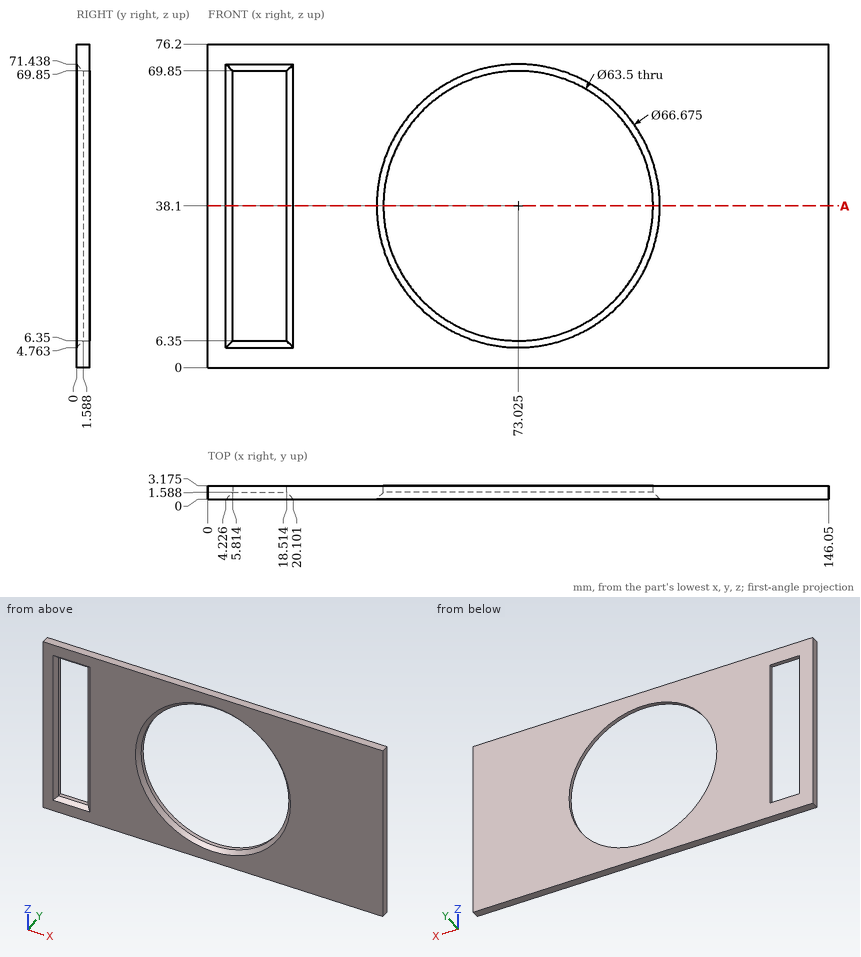
Answer from the drawing. Dimensions are ordinates in mm from the lowest x, y and z of the part. Coordinates: 2 decimals unless noted, no trailing zeros.
1) Section A-A (z = 38.1) is taken. Give the number of separate pieces and of enclosed holes in the cut face, plus the area to 3 significant figures.
Results:
separate pieces: 3
enclosed holes: 0
area: 217 mm2
2) Consider probe 1 along Z at (x, y) = (97, 0.35) (1 decimal); probe 2 along Z at (x, y) = (80.5, 2.6); probe 3 along Y at (x, z) = (104.5, 28) (1 decimal). Determine where each line is inside the solid, lowest interval first.
Results:
probe 1: z = 0 to 15.4, 60.8 to 76.2
probe 2: z = 0 to 7.24, 68.96 to 76.2
probe 3: y = 0.3 to 3.2
3) Flat-ended cylindrical pins translate along their axes: pin 1 (0.8 mm diameter, centred on y = 2.5, z = 24.5, fed in from -X); pin 2 (8 mm diameter, centred on x = 68, z = 13, fed in from -Y). Find the tip coordinate at first contact, or state that the pin passes through.
Results:
pin 1: stops at x = 0
pin 2: passes through
